```python
from build123d import *

# Parameters (mm, degrees)
CLONE2D011_W = 380
CLONE2D011_H = 389
PAD_DEPTH    = 19
SKETCH_W     = 230
SKETCH_H     = 239
POCKET_DEPTH = 19.001


with BuildPart() as part:
    # Clone2D011 → Pad (new body)
    with BuildSketch(Plane.XZ):
        with Locations((190, 194.5)):
            Rectangle(CLONE2D011_W, CLONE2D011_H)
    extrude(amount=PAD_DEPTH)

    # Clone2D010 → Revolution006 (revolve)
    with BuildSketch(Plane(origin=(40, -19, 40), x_dir=(1, 0, 0), z_dir=(0, 0, 1))):
        with BuildLine():
            Line((0, 0), (0, -20))
            add(Edge.make_bspline(
                [(0, -20), (-18, -20), (-18, -9.133286), (-4.506424, -9.133286), (-7.5, 0)],
                knots=[0, 0, 0, 0, 0.5, 1, 1, 1, 1], degree=3, weights=[7, 6.116989, 5.810816, 6.060123, 5.999522]))
            Line((-7.5, 0), (0, 0))
        make_face()
    revolve(axis=Axis((40, -19, 40), (0, 1, 0)))

    # Sketch (on Face5 of Revolution006) → Pocket (cut, through all)
    with BuildSketch(Plane.XZ.offset(19)):
        with Locations((190, 194.5)):
            Rectangle(SKETCH_W, SKETCH_H)
    extrude(amount=-POCKET_DEPTH, mode=Mode.SUBTRACT)


with BuildPart() as part_1:
    # Body placement: moved
    add(part.part.moved(Location((395.5, 0, 899))))


with BuildPart() as part_2:
    # Clone002 placement: moved
    add(part_1.part.moved(Location((-395.5, 0, -899))))


with BuildPart() as part_3:
    # Body016 placement: moved
    add(part_2.part.moved(Location((1170, 0, 899))))


solid = part_3.part
```
Can you work these out from the model? Positions are in its coordinate system, mm. A direction names the side the tool comes from. Round coordinates to 2 decimals unless told otherwise and drop trailing zeros. Order: outer loops, then holes, each group sorted by start corner. A loop starts at its lowest first (then second) coordinate and runs counter-clockwise, first axis right, second up.
(1) On a 3-axis mill with a long thin cutter (end or side, diameter ignored), from which of +Z, -Z, +X, -X, +Y, -Y can I reach the whole of each face in a straight line? I mean faces 4 (the face through (1358, -10, 974)), 5 (the face through (1170, -9, 1091)). Say none if no direction works.
Results are:
face 4: +Y, -Y
face 5: +Z, -Z, -X, +Y, -Y
(2) I'm going to push flat-ended pins straight in: pin 1 (6 mm diameter, centred on x = 1509, z = 1039.5, fed in from -Y); pin 2 (10 mm diameter, centred on x = 1326, z = 983, fed in from +Y). Where does each tip first touch, or does it pass through?
Results are:
pin 1: stops at y = -19
pin 2: passes through
(3) If we section it at C-C (z = 1100.5): Please give me the cut outline in (x, y).
Results are:
outline: (1170, -19) - (1245, -19) - (1245, 0) - (1170, 0) - close; (1475, -19) - (1550, -19) - (1550, 0) - (1475, 0) - close
(4) We'd pull the mould along Z, two halves only. Please class faces 1 (the face through (1357, -9, 1288)), 2 (the face through (1358, -10, 1213)), 3 (the face through (1231, 0, 1096)): +Z half, -Z half, draft (parallel to the pull), parting line (faces both ways), or undercut.
Results are:
face 1: +Z half
face 2: undercut
face 3: draft
(5) If we section it at B-B (y = -13): Please give me the cut outline in (x, z).
Results are:
outline: (1170, 899) - (1550, 899) - (1550, 1288) - (1170, 1288) - close; hole (1245, 974) - (1475, 974) - (1475, 1213) - (1245, 1213) - close
(6) If I drill on L1, parallel to X at y = -10, z = 1163; L2, parallel to Y at x = 1360, z = 1250; L3, parallel to Z at x = 1408, y = -16, over which ranges is the centre line in solid material (lowest first)?
Results are:
L1: x = 1170 to 1245, 1475 to 1550
L2: y = -19 to 0
L3: z = 899 to 974, 1213 to 1288
(7) If we section it at D-D (x = 1506): Please give me the cut outline in (y, z), plus the area to 3 significant figures.
Results are:
outline: (-19, 899) - (0, 899) - (0, 1288) - (-19, 1288) - close
area: 7,390 mm2
(8) If we section it at A-A (x = 1260.5): Please give me the cut outline in (y, z).
Results are:
outline: (-19, 899) - (0, 899) - (0, 974) - (-19, 974) - close; (-19, 1213) - (0, 1213) - (0, 1288) - (-19, 1288) - close
